Autodesk Inventor part; units mm, degrees
ref_plane "Work Plane5" through (-24.85, -3.5, 5) normal (0, 0, 1) x (1, 0, 0)
ref_plane "YZ Plane" through (0, 0, 0) normal (1, 0, 0) x (0, 1, 0)
ref_plane "XZ Plane" through (0, 0, 0) normal (0, 1, 0) x (-1, 0, 0)
ref_plane "Work Plane5" through (-24.85, -3.5, 5) normal (0, 0, 1) x (1, 0, 0)
sketch "Sketch16" plane through (-24.85, -3.5, 5) normal (0, 0, 1) x (1, 0, 0)
  circle A0 centre (0, 0) radius 6.5 construction
  arc A1 (-8.312, 5) -> (8.312, 5) centre (0, 0) ccw
  line L0 (9.7, 0) -> (-9.7, 0) construction
  line L1 (8.312, 5) -> (-8.312, 5)
  arc A2 (-4.3933, 4.9254) -> (4.3933, 4.9254) centre (0, 0) ccw
  arc A3 (-4.3081, 5) -> (4.3081, 5) centre (0, 0) ccw
  point P0 (24.85, 3.5)
  point P1 (4.4598, 5)
  point P2 (-4.4598, 5)
  dimension "d45" = 5
extrude "Extrusion16" add sketch "Sketch16" against normal blind 5 contours L1 A3 A2 A1
sketch "Sketch17" plane through (-24.85, -3.5, 5) normal (0, 0, 1) x (1, 0, 0)
  circle A0 centre (-21.25, -15.25) radius 2.15
  circle A1 centre (21.25, -15.25) radius 2.15
  arc A2 (-24.25, -6.25) -> (-26.25, -8.25) centre (-24.25, -8.25) ccw
  line L0 (-23.35, -6.25) -> (-24.25, -6.25)
  arc A3 (-23.35, -6.25) -> (-21.35, -4.25) centre (-23.35, -4.25) ccw
  line L1 (-21.35, -0.6245) -> (-21.35, -4.25)
  arc A4 (-21.35, -0.6245) -> (-21.35, 0.6245) centre (-19.45, 0) ccw
  line L2 (-21.35, 4.25) -> (-21.35, 0.6245)
  arc A5 (-19.35, 6.25) -> (-21.35, 4.25) centre (-19.35, 4.25) ccw
  line L3 (-19.35, 6.25) -> (-16.95, 6.25)
  line L4 (-16.95, 6.25) -> (-16.95, -6.25)
  line L5 (-16.95, -6.25) -> (6.65, -6.25)
  line L6 (6.65, -6.25) -> (6.65, 6.25)
  line L7 (6.65, 6.25) -> (9.05, 6.25)
  arc A6 (11.05, 4.25) -> (9.05, 6.25) centre (9.05, 4.25) ccw
  line L8 (11.05, 4.25) -> (11.05, 0.6245)
  arc A7 (11.05, 0.6245) -> (11.05, -0.6245) centre (9.15, 0) ccw
  line L9 (11.05, -0.6245) -> (11.05, -4.25)
  arc A8 (11.05, -4.25) -> (13.05, -6.25) centre (13.05, -4.25) ccw
  line L10 (13.05, -6.25) -> (24.25, -6.25)
  arc A9 (26.25, -8.25) -> (24.25, -6.25) centre (24.25, -8.25) ccw
  line L11 (26.25, -8.25) -> (26.25, -20.25)
  arc A10 (16.25, -12.25) -> (14.25, -10.25) centre (14.25, -12.25) ccw
  line L12 (14.25, -10.25) -> (-14.25, -10.25)
  arc A11 (-14.25, -10.25) -> (-16.25, -12.25) centre (-14.25, -12.25) ccw
  line L13 (-26.25, -20.25) -> (-26.25, -8.25)
  line L14 (-16.25, -12.25) -> (-16.25, -20.25)
  line L15 (-26.25, -20.25) -> (-16.25, -20.25)
  line L16 (16.25, -20.25) -> (26.25, -20.25)
  line L17 (16.25, -12.25) -> (16.25, -20.25)
  point P0 (24.85, 3.5)
extrude "Extrusion17" add sketch "Sketch17" against normal blind 5
sketch "Sketch18" plane through (-24.85, -3.5, 0) normal (0, 0, -1) x (-1, 0, 0)
  line L0 (16.95, -6.25) -> (7.4181, -6.25)
  line L1 (14.25, -6.25) -> (26.25, -6.25)
  line L2 (26.25, -6.25) -> (26.25, 6.25)
  line L3 (26.25, 6.25) -> (14.25, 6.25)
  line L4 (14.25, 6.25) -> (14.25, -6.25)
  point P0 (-24.85, 3.5)
extrude "Extrusion18" cut sketch "Sketch18" against normal blind 5
sketch "Sketch19" plane through (-24.85, -3.5, 0) normal (0, 0, -1) x (-1, 0, 0)
  line L0 (-4.4598, 5) -> (-15.1519, 5)
  line L1 (-15.1519, 5) -> (-15.1519, 7.7901)
  line L2 (-15.1519, 7.7901) -> (-4.4598, 7.7901)
  line L3 (-4.4598, 7.7901) -> (-4.4598, 5)
  point P0 (-24.85, 3.5)
extrude "Extrusion19" cut sketch "Sketch19" against normal blind 5
sketch "Sketch20" plane through (-24.85, -3.5, 0) normal (0, 0, -1) x (-1, 0, 0)
  line L0 (-4.3081, 5) -> (-10.904, 5)
  arc A0 (-13.05, -6.25) -> (-11.05, -4.25) centre (-13.05, -4.25) ccw
  line L1 (-14.25, -10.25) -> (14.25, -10.25)
  line L2 (24.25, -6.25) -> (7.4181, -6.25)
  line L3 (8.312, 5) -> (4.3081, 5)
  line L4 (-6.65, -0.817) -> (-6.65, 0.817)
  arc A1 (-4.4598, 5) -> (-6.65, 0.817) centre (0, 0) ccw
  line L5 (-7.14, 5) -> (-12.1327, 5)
  line L6 (-13.05, -6.25) -> (-7.4181, -6.25)
  arc A2 (-8.1939, -10.25) -> (11.5386, -6.25) centre (0, 0) ccw
  arc A3 (-12.1327, 5) -> (-11.5386, -6.25) centre (0, 0) ccw
  arc A4 (7.4181, -6.25) -> (8.312, 5) centre (0, 0) ccw
  arc A5 (-8.312, 5) -> (-7.4181, -6.25) centre (0, 0) ccw
  point P0 (4.4598, 5)
  point P1 (-24.85, 3.5)
extrude "Extrusion20" cut sketch "Sketch20" against normal blind 5 contours A5 L6 A3 L5 L0
sketch "Sketch21" plane through (-24.85, -3.5, 0) normal (0, 0, -1) x (-1, 0, 0)
  line L0 (-13.05, -6.25) -> (-24.25, -6.25)
  line L1 (-15.1128, -6.25) -> (-9.6695, -6.25)
  line L2 (-9.6695, -6.25) -> (-9.6695, -4.6771)
  line L3 (-9.6695, -4.6771) -> (-15.1128, -4.6771)
  line L4 (-15.1128, -4.6771) -> (-15.1128, -6.25)
  point P0 (-24.85, 3.5)
extrude "Extrusion21" cut sketch "Sketch21" against normal blind 5
fillet "Fillet2" radius 2 4 edges at (-17.4319, -9.75, 2.5) (-33.162, 1.5, 2.5) (-16.538, 1.5, 2.5) (-32.2681, -9.75, 2.5)
sketch "Sketch22" plane through (-24.85, -3.5, 0) normal (0, 0, -1) x (-1, 0, 0)
  line L0 (7.0915, 5) -> (4.3081, 5)
  line L1 (2.1207, -6.25) -> (-2.1207, -6.25)
  line L2 (-6.65, -0.817) -> (-6.65, 0.817)
  line L3 (-2.414, -6.25) -> (2.414, -6.25)
  arc A0 (-4.3081, 5) -> (-2.1207, -6.25) centre (0, 0) ccw construction
  arc A1 (2.1207, -6.25) -> (4.3081, 5) centre (0, 0) ccw construction
  arc A2 (-2.1207, -6.25) -> (2.1207, -6.25) centre (0, 0) ccw
  point P0 (4.4598, 5)
  point P1 (-24.85, 3.5)
extrude "Extrusion23" cut sketch "Sketch22" against normal blind 5
properties part number "BearingSupport"
CAD build for the part. Positions are in the model's coordinates, mm. A direction names the side the tool comes from. Give positions to 0.01 mm unless a question says otherwise; leave off trailing zeros. Order: outer loops, then holes, each group sorted by start corner. A loop starts at its lowest first (then second) coordinate and runs counter-clockwise, first axis right, second up.
(1) Saw through at C-C, the plane x = -7. Give the cut face in (y, z), then the cut area to 3 significant figures.
(2) Saw through at D-D, the plane x = -17. Give the cut face in (y, z).
(3) Saw through at B-B, the plane z = 2.35. Give the cut face in (x, y).
(4) Drill centre lines: L1, parallel to X at y = -19.75, z = 3.5; L2, parallel to X at y = -3.25, z = 0.7; L3, parallel to X at y = -20.5, z = 4.5. Where is each one in solid material? Low to high.
(5) Saw through at A-A, the plane x = -46.1. Give the cut face in (y, z).
(6) Tool access for faces 5 (the flat face through (-8.6, -20, 3)), 6 (the flat face through (-43, -9.75, 3)), 7 (the cylindrical face through (-18.4, -4.9, 2.5)): list every direction of +Z, -Z, +X, -X, +Y, -Y with a clear straight run to the whole face (end or side of a thin tool).
(7) Mould opens along X. For faces 1 (the cylindrical face through (-34.115, -8.901, 2.535)), 2 (the flat face through (1.4, -18, 3)), 3 (the cylindrical face through (-40.5, -14.32, 2.54)), 4 (the flat face through (-31, 1.5, 3)) say: released by +X, released by -X, zero draft, split by the parting line, or undercut.
(8) Flat gauge pins, fed straight in: pin 1 (1.5 mm diameter, centred on x = -20.5, z = 0.5, fed in from -Y); pin 2 (3 mm diameter, centred on y = -8.5, z = 2.5, fed in from -X); pin 3 (1.5 mm diameter, centred on y = -5.5, z = 4.5, fed in from +X). Where does each tip first touch, or does it go through?
Results found:
1. outline: (-23.75, 0) - (-9.75, 0) - (-9.75, 5) - (-23.75, 5) - close
1. area: 70.0 mm2
2. outline: (-13.75, 0) - (1.35, 0) - (1.35, 5) - (-13.75, 5) - close
3. outline: (-51.1, -23.75) - (-41.1, -23.75) - (-41.1, -15.75) arc R2 cw to (-39.1, -13.75) - (-10.6, -13.75) arc R2 cw to (-8.6, -15.75) - (-8.6, -23.75) - (1.4, -23.75) - (1.4, -11.75) arc R2 ccw to (-0.6, -9.75) - (-13.95, -9.75) arc R2 cw to (-15.81, -7.02) arc R9.7 ccw to (-15.35, -5.47) arc R9.7 ccw to (-15.35, -1.53) arc R9.7 ccw to (-15.92, 0.28) arc R2 ccw to (-17.76, 1.5) - (-20.54, 1.5) arc R6.6 cw (long way) to (-29.16, 1.5) - (-31.94, 1.5) arc R2 ccw to (-33.78, 0.28) arc R9.7 ccw to (-33.89, -7.02) arc R2 cw to (-35.75, -9.75) - (-49.1, -9.75) arc R2 ccw to (-51.1, -11.75) - close; hole circle Ø4.3 at (-46.1, -18.75); hole circle Ø4.3 at (-3.6, -18.75)
4. L1: x = -51.1 to -48, -44.2 to -41.1, -8.6 to -5.5, -1.7 to 1.4
4. L2: x = -34.55 to -31.45, -18.25 to -15.15
4. L3: x = -51.1 to -47.35, -44.85 to -41.1, -8.6 to -4.85, -2.35 to 1.4
5. outline: (-23.75, 0) - (-20.9, 0) - (-20.9, 5) - (-23.75, 5) - close; (-16.6, 0) - (-9.75, 0) - (-9.75, 5) - (-16.6, 5) - close
6. face 5: +Z, -Z, -Y
6. face 6: +Z, -Z, -X, +Y
6. face 7: +Z, -Z
7. face 1: released by -X
7. face 2: released by +X
7. face 3: undercut
7. face 4: zero draft
8. pin 1: stops at y = -13.75
8. pin 2: stops at x = -50.07
8. pin 3: stops at x = -15.23
